Geometry: see drawing. Coordinates: mm, zero at the bounding-box minimum. A direction names the side the tool comes from. Round coordinates to 2 decimals unless told otherwise and drop trailing zeros. Order: outer loops, then holes, each group sorted by start corner. A loop starts at its lowest first (then second) coordinate and runs counter-clockwise, first axis right, second up. Notation, with made-up numbers: (-31.75, 73) -> (1.25, 73) arc R19 ccw to (1.25, 82) -> close; hole circle Ø1 at (85.25, -25). An arc over 180 degrees is marked (long way). Use a Markdown table: item, result.
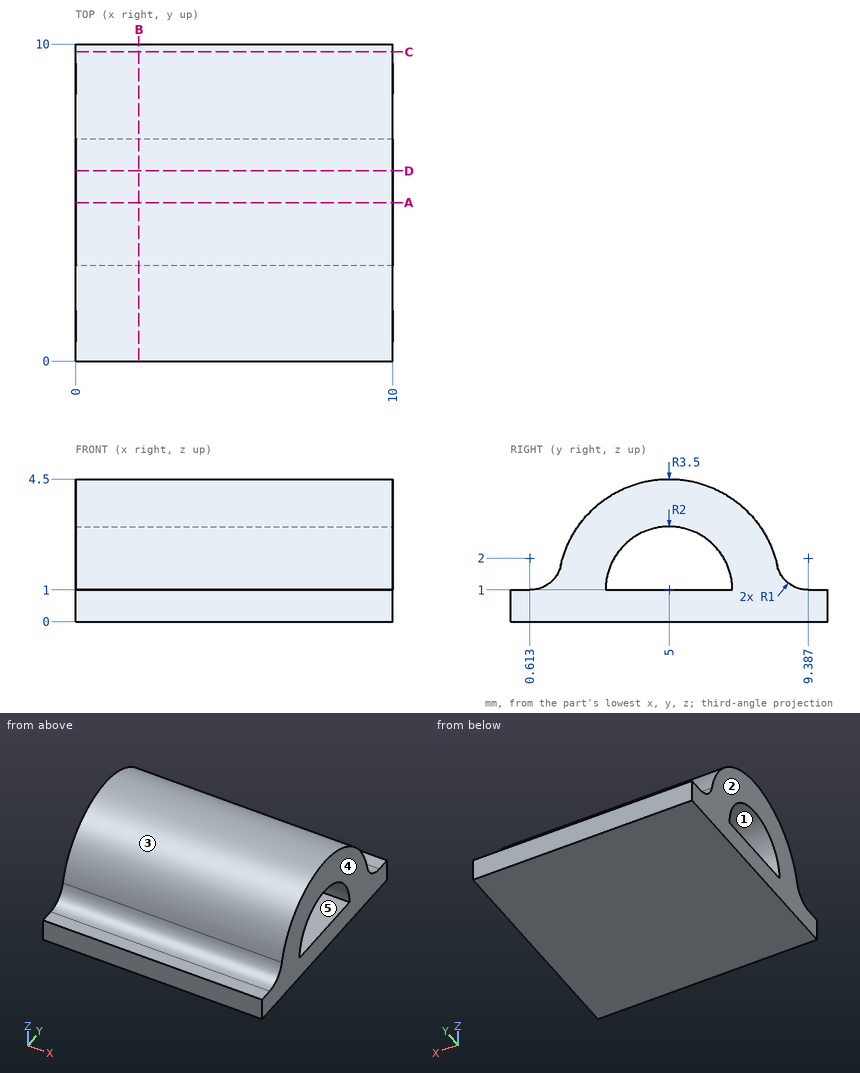
1) Cut plane A-A on y = 5. Return loops of the section in (x, z), and give its area (3 significant figures).
Answer key:
| item | result |
|---|---|
| outline | (0, 0) -> (10, 0) -> (10, 1) -> (0, 1) -> close; (0, 3) -> (10, 3) -> (10, 4.5) -> (0, 4.5) -> close |
| area | 25.0 mm^2 |
2) Draft query along Y for the marked faces 3, 4 and 5. Return one class per face: released by +Y, released by -Y, zero draft, split by the parting line, or undercut.
Answer key:
| item | result |
|---|---|
| face 3 | split by the parting line |
| face 4 | zero draft |
| face 5 | undercut |
3) Cut plane D-D on y = 6. Return loops of the section in (x, z) (1 decimal).
Answer key:
| item | result |
|---|---|
| outline | (0, 0) -> (10, 0) -> (10, 1) -> (0, 1) -> close; (0, 2.7) -> (10, 2.7) -> (10, 4.4) -> (0, 4.4) -> close |
4) Cut plane C-C on y = 9.75. Return loops of the section in (x, z).
Answer key:
| item | result |
|---|---|
| outline | (0, 0) -> (10, 0) -> (10, 1) -> (0, 1) -> close |
5) Set-up query: the marked faces 1 and 2. Return all of +Z, -Z, +X, -X, +Y, -Y with unobstructed straight access to the full face (end or side cutting, diameter ignored); none if empty.
Answer key:
| item | result |
|---|---|
| face 1 | +X, -X |
| face 2 | +Z, -Z, -X, +Y, -Y |
6) Cut plane B-B on x = 2. Return loops of the section in (y, z).
Answer key:
| item | result |
|---|---|
| outline | (0, 0) -> (10, 0) -> (10, 1) -> (9.39, 1) arc R1 cw to (8.41, 1.78) arc R3.5 ccw to (1.59, 1.78) arc R1 cw to (0.61, 1) -> (0, 1) -> close; hole (3, 1) -> (7, 1) arc R2 ccw to start |
7) Ray query, probe 1 along Z at (x, y) = (5.5, 5); probe 2 along Y at (x, z) = (4.5, 1.55) (1 decimal); probe 3 along Z at (x, y) = (2, 3.25) (1 decimal). Return the intervals inside material, ascending.
Answer key:
| item | result |
|---|---|
| probe 1 | z = 0 to 1, 3 to 4.5 |
| probe 2 | y = 1.5 to 3.1, 6.9 to 8.5 |
| probe 3 | z = 0 to 1, 2 to 4 |
8) Contact query for a flat-ended pin moving along its axis: P1, Ø1.5, axis at x = 3.5, z = 3, coming from the +Y side. Output: stop coordinate, or through.
Answer key:
| item | result |
|---|---|
| P1 | stops at y = 8.27 |
